Could you check a few things on this model? Use its own coordinates, in mm. Face numbers are marked on the shaded views. A direction names the side the tool comes from. Coordinates: 2 decimals unless noted, no trailing zeros. Write each loop counter-clockwise with the first axis right and the second up, starting at its lowest first coordinate (ties: lowest second). Pieces come first, ordered by that corner, then holes.
Item 1: I want a section at D-D on z = 31.5. Please give me the cut outline in (x, y), then the cut area to 3 significant figures.
Item 2: Thinking about a two-plate mould opening in Y: for the marked faces 1, 2 and 3, which applies, +Y half, -Y half, draft (parallel to the pull), parting line (faces both ways), or undercut?
Item 3: If I drill on probe 1 along Z at (x, y) = (-1, 4); probe 2 along X at (y, z) = (-14.5, 1); probe 3 along Y at (x, z) = (-13, 13), over which ranges is the centre line in solid material (lowest first)?
Item 4: I want a section at A-A on x = -13. Please give me the cut outline in (y, z).
Item 5: I want a section at C-C on y = 11. Please give me the cut outline in (x, z), then the cut area to 3 significant figures.
Item 6: Which directions (+Z, -Z, +X, -X, +Y, -Y) give clear straight access to the entire face, cutting with the end or side of a thin tool? Please do the marked faces 4, 5 and 6.
Item 7: For P1, Ø17, axis at x = 25, z = 40, coming from the +Y side; P2, Ø2.5, axis at y = 1, z = 7.5, coming from the +X side; P3, Ø2, axis at y = 10.5, z = 35, coming from the -X side; P4, Ø24.5, axis at x = 18, z = 33.5, coming from the +Y side, each with a flat end and sliding along its axis, tell me the tip position at first contact or that it passes through.
Item 8: I want a section at B-B on y = -12.5. Please give me the cut outline in (x, z).
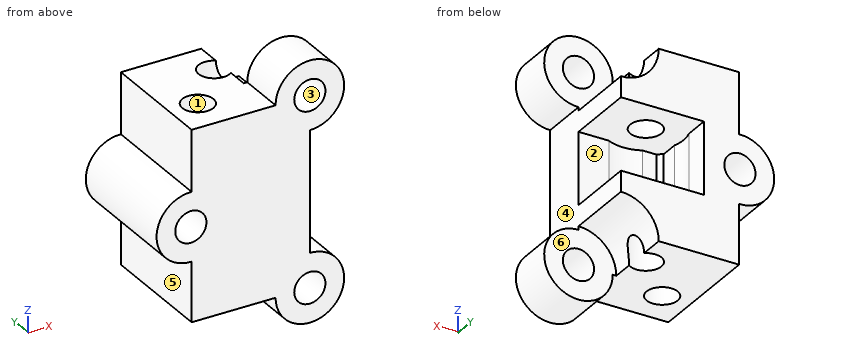
from build123d import *

# Parameters (mm, degrees)
F1_DEPTH       = 25
F3_D           = 13.2
F3_CBORE_D     = 19.25
F3_CBORE_DEPTH = 0
F5_D           = 13.2
F5_CBORE_D     = 19.25
F5_CBORE_DEPTH = 0
F6_W           = 40
F6_H           = 30.5
F7_DEPTH       = 30
F8_R           = 16
F9_DEPTH       = 30.5
F10_R          = 16
F11_DEPTH      = 30


with BuildPart() as f1:
    # F0 (on Front) → F1 (new body, symmetric)
    with BuildSketch(Plane.XZ):
        with BuildLine():
            Line((25, -25.5), (25, -40))
            Line((25, -40), (10.5, -40))
            ThreePointArc((10.5, -40), (25, -54.5), (39.5, -40))
            ThreePointArc((39.5, -40), (35.2530483272, -29.7469516728), (25, -25.5))
        make_face()
        with BuildLine():
            Line((10.5, -40), (25, -40))
            Line((25, -40), (25, -25.5))
            ThreePointArc((25, -25.5), (14.7469516728, -29.7469516728), (10.5, -40))
        make_face()
        with BuildLine():
            Line((-25, -40), (10.5, -40))
            ThreePointArc((10.5, -40), (14.7469516728, -29.7469516728), (25, -25.5))
            Line((25, -25.5), (25, 25.5))
            ThreePointArc((25, 25.5), (14.7469516728, 29.7469516728), (10.5, 40))
            Line((10.5, 40), (-25, 40))
            Line((-25, 40), (-25, 14.2162181315))
            ThreePointArc((-25, 14.2162181315), (-14.9640357801, 9.8540823977), (-10.8347666082, -0.279916916))
            ThreePointArc((-10.8347666082, -0.279916916), (-14.9640357801, -10.4139162298), (-25, -14.7760519636))
            Line((-25, -14.7760519636), (-25, -40))
        make_face()
        with BuildLine():
            ThreePointArc((10.5, 40), (14.7469516728, 29.7469516728), (25, 25.5))
            Line((25, 25.5), (25, 40))
            Line((25, 40), (10.5, 40))
        make_face()
        with BuildLine():
            Line((25, 40), (25, 25.5))
            ThreePointArc((25, 25.5), (35.2530483272, 29.7469516728), (39.5, 40))
            ThreePointArc((39.5, 40), (25, 54.5), (10.5, 40))
            Line((10.5, 40), (25, 40))
        make_face()
        with BuildLine():
            ThreePointArc((-25, 14.2162181315), (-39.8347666082, -0.279916916), (-25, -14.7760519636))
            Line((-25, -14.7760519636), (-25, 14.2162181315))
        make_face()
        with BuildLine():
            Line((-25, 14.2162181315), (-25, -14.7760519636))
            ThreePointArc((-25, -14.7760519636), (-14.9640357801, -10.4139162298), (-10.8347666082, -0.279916916))
            ThreePointArc((-10.8347666082, -0.279916916), (-14.9640357801, 9.8540823977), (-25, 14.2162181315))
        make_face()
    extrude(amount=F1_DEPTH, both=True)

    # F3 (through all)
    with Locations(Plane.XZ.offset(25)):
        with Locations((25, 40), (-25.3347666082, -0.279916916), (25, -40)):
            CounterBoreHole(F3_D / 2, F3_CBORE_D / 2, F3_CBORE_DEPTH)

    # F5 (through all)
    with Locations(Plane.XY.offset(40)):
        with Locations((-13, -9.3407420599), (5.0832007976, 9.3407420599)):
            CounterBoreHole(F5_D / 2, F5_CBORE_D / 2, F5_CBORE_DEPTH)

    # F6 (on face) → F7 (cut)
    with BuildSketch(Plane(origin=(0, 25, 0), x_dir=(-1, 0, 0), z_dir=(0, 1, 0))):
        with Locations((-9.9, 0)):
            Rectangle(F6_W, F6_H)
    extrude(amount=-F7_DEPTH, mode=Mode.SUBTRACT)

    # F8 (on face) → F9 (cut)
    with BuildSketch(Plane.XY.offset(-15.25)):
        with Locations((5.0832007976, 9.3407420599)):
            Circle(F8_R)
    extrude(amount=F9_DEPTH, mode=Mode.SUBTRACT)

    # F10 (on face) → F11 (cut)
    with BuildSketch(Plane(origin=(0, 25, 0), x_dir=(-1, 0, 0), z_dir=(0, 1, 0))):
        with Locations((-25, 40)):
            Circle(F10_R)
        with Locations((-25, -40)):
            Circle(F10_R)
    extrude(amount=-F11_DEPTH, mode=Mode.SUBTRACT)


solid = f1.part
Response values:
1. outline: (-25, -25) - (36.75, -25) - (36.75, -5) - (11.44, -5) - (11.44, 7.58) arc R6.6 cw (long way) to (11.44, 11.1) - (11.44, 25) - (-25, 25) - close; hole circle Ø13.2 at (-13, -9.34)
1. area: 2,060 mm2
2. face 1: undercut
2. face 2: +Y half
2. face 3: draft
3. probe 1: z = -40 to -15.25, 15.25 to 40
3. probe 2: x = -39.78 to -31.81, -18.86 to -17.12, -8.88 to 25
3. probe 3: y = -25 to -15.94, -2.74 to 25
4. outline: (-25, -40) - (-15.94, -40) - (-15.94, 40) - (-25, 40) - close; (-2.74, -40) - (25, -40) - (25, 40) - (-2.74, 40) - close
5. outline: (-25, -40) - (-1.3, -40) - (-1.3, -15.25) - (-10.83, -15.25) - (-10.83, 15.25) - (-1.3, 15.25) - (-1.3, 40) - (-25, 40) - (-25, 14.22) arc R14.5 ccw (long way) to (-25, -14.78) - close; (11.47, -31.46) arc R16 cw to (25, -24) - (25, -15.25) - (11.47, -15.25) - close; (11.47, 15.25) - (25, 15.25) - (25, 24) arc R16 cw to (11.47, 31.46) - close; hole circle Ø13.2 at (-25.33, -0.28)
5. area: 2,100 mm2
6. face 4: +X, +Y, -Y
6. face 5: -Z, -X, +Y, -Y
6. face 6: -Z, +X, +Y
7. P1: stops at y = -5
7. P2: stops at x = -10.1
7. P3: stops at x = -25
7. P4: stops at y = 25
8. outline: (-25, -40) - (-18.79, -40) - (-18.79, -1.17) arc R6.6 cw (long way) to (-18.79, 0.61) - (-18.79, 40) - (-25, 40) - (-25, 14.22) arc R14.5 ccw (long way) to (-25, -14.78) - close; (-7.21, -40) - (10.5, -40) arc R14.5 ccw (long way) to (25, -25.5) - (25, 25.5) arc R14.5 ccw (long way) to (10.5, 40) - (-7.21, 40) - close; hole circle Ø13.2 at (25, -40); hole circle Ø13.2 at (25, 40)
